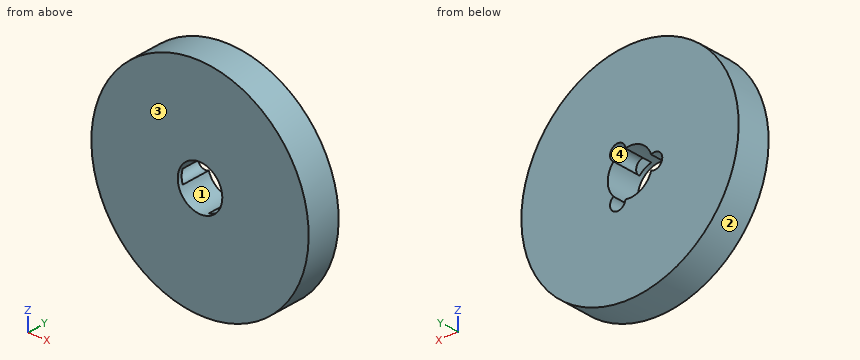
from build123d import *

# Parameters (mm, degrees)
SKETCH1_R           = 97.5
BOSS_EXTRUDE1_DEPTH = 30
SKETCH2_R           = 20
CUT_EXTRUDE1_DEPTH  = 142.111657917
SKETCH3_R           = 6.867943311
CUT_EXTRUDE2_DEPTH  = 26.109463
CIRPATTERN1_START   = 3.890536695
CIRPATTERN1_DEPTH   = 26.109463305


# Read off the part's stored shape, not the designer's step: CirPattern1
with BuildPart() as part:
    # Sketch1 → Boss-Extrude1 (new body)
    with BuildSketch(Plane(origin=(0, 0, 0), x_dir=(1, 0, 0), z_dir=(0, 1, 0))):
        with Locations(Location((0, 0, 0), (0, 0, 270))):
            Circle(SKETCH1_R)
    extrude(amount=BOSS_EXTRUDE1_DEPTH)

    # Sketch2 → Cut-Extrude1 (cut, through all)
    with BuildSketch(Plane(origin=(0, 0, 0), x_dir=(1, 0, 0), z_dir=(0, 1, 0))):
        with Locations(Location((0, 0, 0), (0, 0, 270))):
            Circle(SKETCH2_R)
    extrude(amount=CUT_EXTRUDE1_DEPTH, mode=Mode.SUBTRACT)

    # Sketch3 → Cut-Extrude2 (cut)
    with BuildSketch(Plane(origin=(0, 30, 0), x_dir=(1, 0, 0), z_dir=(0, 1, 0))):
        with Locations((-22.081174807, 0)):
            Circle(SKETCH3_R)
    extrude(amount=-CUT_EXTRUDE2_DEPTH, mode=Mode.SUBTRACT)

    # CirPattern1 outline → CirPattern1 (cut)
    with BuildSketch(Plane(origin=(0, 0, 0), x_dir=(1, 0, 0), z_dir=(0, 1, 0)).offset(CIRPATTERN1_START)):
        with BuildLine():
            ThreePointArc((4.186376244, 19.556948994), (10, 17.320508076), (14.843626527, 13.403982674))
            ThreePointArc((14.843626527, 13.403982674), (14.474559059, 25.070671708), (4.186376244, 19.556948994))
        make_face()
        with BuildLine():
            ThreePointArc((14.843626527, -13.403982674), (10, -17.320508076), (4.186376244, -19.556948994))
            ThreePointArc((4.186376244, -19.556948994), (14.474559059, -25.070671708), (14.843626527, -13.403982674))
        make_face()
    extrude(amount=CIRPATTERN1_DEPTH, mode=Mode.SUBTRACT)


solid = part.part
Part model, mm, in its own coordinate system. Face numbers are marked on the shaded views. Round coordinates to 2 decimals unless told otherwise and drop trailing zeros. Write each loop counter-clockwise with the first axis right and the second up, starting at its lowest first coordinate (ties: lowest second). Pieces come first, ordered by that corner, then holes. Notation, with made-up numbers: (28, -7) - (81, -7) arc R35 ccw to (81, 29) - close; hole circle Ø3 at (-23, 78). An arc over 180 degrees is marked (long way). Use CSV: the item, a comma, the result in double quotes.
Item 1: Slice it at B-B, the plane x = 0. Write the cut outline in (y, z), then the cut area to 3 significant figures.
Results list:
outline,"(0, -97.5) - (30, -97.5) - (30, -20) - (0, -20) - close; (0, 20) - (30, 20) - (30, 97.5) - (0, 97.5) - close"
area,"4,650 mm²"
Item 2: Slice it at C-C, the plane y = 20.25. Write the cut outline in (x, z), then the cut area to 3 significant figures.
Results list:
outline,"circle Ø195 at (0, 0); hole (-19.03, -6.15) arc R20 ccw to (4.19, -19.56) arc R6.87 ccw (long way) to (14.84, -13.4) arc R20 ccw to (14.84, 13.4) arc R6.87 ccw (long way) to (4.19, 19.56) arc R20 ccw to (-19.03, 6.15) arc R6.87 ccw (long way) to start"
area,"28,300 mm²"
Item 3: Pull direction Z, two halves, no side cores. Call the marked faces 1, 2, 3 and 4: pulls with the +Z half, pulls with the -Z half, needs draft (parallel to the pull), parting line crosses it, or undercut.
Results list:
face 1,"undercut"
face 2,"parting line crosses it"
face 3,"needs draft"
face 4,"undercut"
Item 4: Wall check: L1, parallel to Z at x = 1, y = 24.5; L2, parallel to Z at x = -20, y = 25; L3, parallel to X at y = 6.5, z = 24. Give the ranges that are in metal, low to high.
Results list:
L1,"z = -97.49 to -19.97, 19.97 to 97.49"
L2,"z = -95.43 to -6.55, 6.55 to 95.43"
L3,"x = -94.5 to 6.21, 15.88 to 94.5"
Item 5: Slice it at D-D, the plane z = 67. Write the cut outline in (x, y).
Results list:
outline,"(-70.83, 0) - (70.83, 0) - (70.83, 30) - (-70.83, 30) - close"
Item 6: Flat gauge pins, fed straight in: P1, Ø1, axis at y = 7.5, z = 41, coming from the +X side; P2, Ø10, axis at x = -17.5, y = 5, coming from the +Z side; P3, Ø2, axis at y = 16, z = -47, coming from the +X side. Where does each tip first touch, or does it go through?
Results list:
P1,"stops at x = 88.69"
P2,"stops at z = 96.7"
P3,"stops at x = 85.97"
Item 7: Slice it at A-A, the plane z = 0. Write the cut outline in (x, y).
Results list:
outline,"(-97.5, 0) - (-20, 0) - (-20, 3.89) - (-28.95, 3.89) - (-28.95, 30) - (-97.5, 30) - close; (20, 0) - (97.5, 0) - (97.5, 30) - (20, 30) - close"
